Autodesk Fusion 360 part; units mm, degrees
sketch "Sketch1" plane through (0, 0, 0) normal (0, 0, 1) x (1, 0, 0)
  circle A0 centre (0, 0) radius 4.6
  circle A1 centre (0, 0) radius 2
  line L0 (1.7394, -0.9872) -> (1.7246, 1.0128)
  line L1 (1.7246, 1.0128) -> (-0.0148, 1.9999)
  line L2 (-0.0148, 1.9999) -> (-1.7394, 0.9872)
  line L3 (-1.7394, 0.9872) -> (-1.7246, -1.0128)
  line L4 (-1.7246, -1.0128) -> (0.0148, -1.9999)
  line L5 (0.0148, -1.9999) -> (1.7394, -0.9872)
  dimension "d1" = 9.2
  dimension "d2" = 4
extrude "Extrude1" add sketch "Sketch1" against normal blind 6.5 contours A1 L0 | A1 L1 | L0 L1 L2 L3 L4 L5 | A1 L5 | A1 L2 | A1 L4 | A1 L3 makes body 1
extrude "Extrude2" add sketch "Sketch1" along normal blind 4 separate body contours A0 | A1 L0 | A1 L1 | A1 L5 | A1 L2 | A1 L4 | A1 L3 makes body 2
thread "Thread1" thread offset 0 thread length 10
combine "Combine1" operation add target body 1 tool bodies 2
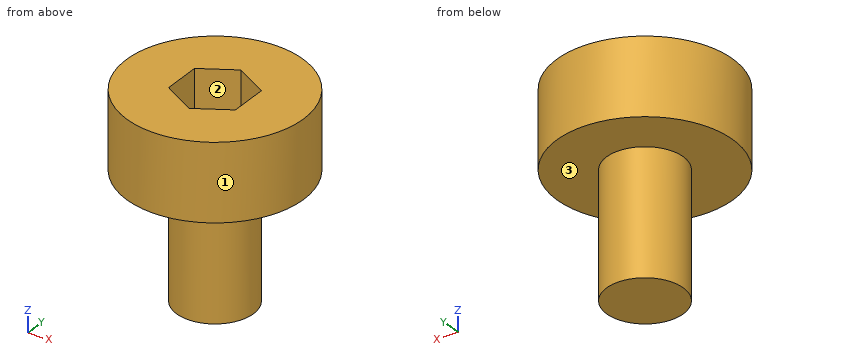
Design review of the part built by this model. Coordinates are the model's own, in mm. Face numbers are marked on the shaded views. A direction names the side the tool comes from. Round coordinates to 2 decimals unless told otherwise and drop trailing zeros. Write each loop counter-clockwise with the first axis right and the second up, starting at its lowest first coordinate (ties: lowest second). Pieces come first, ordered by that corner, then holes.
Item 1: For the marked faces 1, 2 and 3, list the 3-axis set-ups (+Z, -Z, +X, -X, +Y, -Y) from which the entire face can be reached by the end or side of a thin tool; tool diameter is ignored.
Item 2: We need section D-D on x = 3. Write out the cut boundary in (y, z), and give its area (3 significant figures).
Item 3: We need section C-C on z = -1.25. Write out the cut boundary in (x, y).
Item 4: Clearance check with flat-ended pins moving along their axes: pin 1 Ø2 at (x, z) = (-3.5, 1.5) entering from +Y; pin 2 Ø3 at (x, y) = (3.5, 3) entering from -Z; pin 3 Ø1 at (x, z) = (-2.5, 0) entering from -Y. State where each tip first meets the part, or that it passes through.
Item 5: We need section A-A on y = 0.5. Write out the cut boundary in (x, z), and give its area (3 significant figures).
Item 6: For probe 1 along Z at (x, y) = (-0.25, -1.75); probe 2 along Z at (x, y) = (-3.5, -1); probe 3 along X at (y, z) = (1.5, 3), list the stretches that pass through material, from the lowest coordinate up.
Item 7: We need section B-B on x = 0.25. Write out the cut boundary in (y, z).
Returned:
1. face 1: +Z, -Z
1. face 2: +Z
1. face 3: -Z
2. outline: (-3.49, 0) - (3.49, 0) - (3.49, 4) - (-3.49, 4) - close
2. area: 27.9 mm2
3. outline: circle Ø4 at (0, 0)
4. pin 1: stops at y = 3.86
4. pin 2: stops at z = 0
4. pin 3: stops at y = -4.14
5. outline: (-4.57, 0) - (-1.94, 0) - (-1.94, -6.5) - (1.94, -6.5) - (1.94, 0) - (4.57, 0) - (4.57, 4) - (1.73, 4) - (1.73, 0) - (-1.74, 0) - (-1.74, 4) - (-4.57, 4) - close
5. area: 47.9 mm2
6. probe 1: z = -6.5 to 0
6. probe 2: z = 0 to 4
6. probe 3: x = -4.35 to -0.87, 0.87 to 4.35
7. outline: (-4.59, 0) - (-1.98, 0) - (-1.98, -6.5) - (1.98, -6.5) - (1.98, 0) - (4.59, 0) - (4.59, 4) - (1.85, 4) - (1.85, 0) - (-1.86, 0) - (-1.86, 4) - (-4.59, 4) - close
